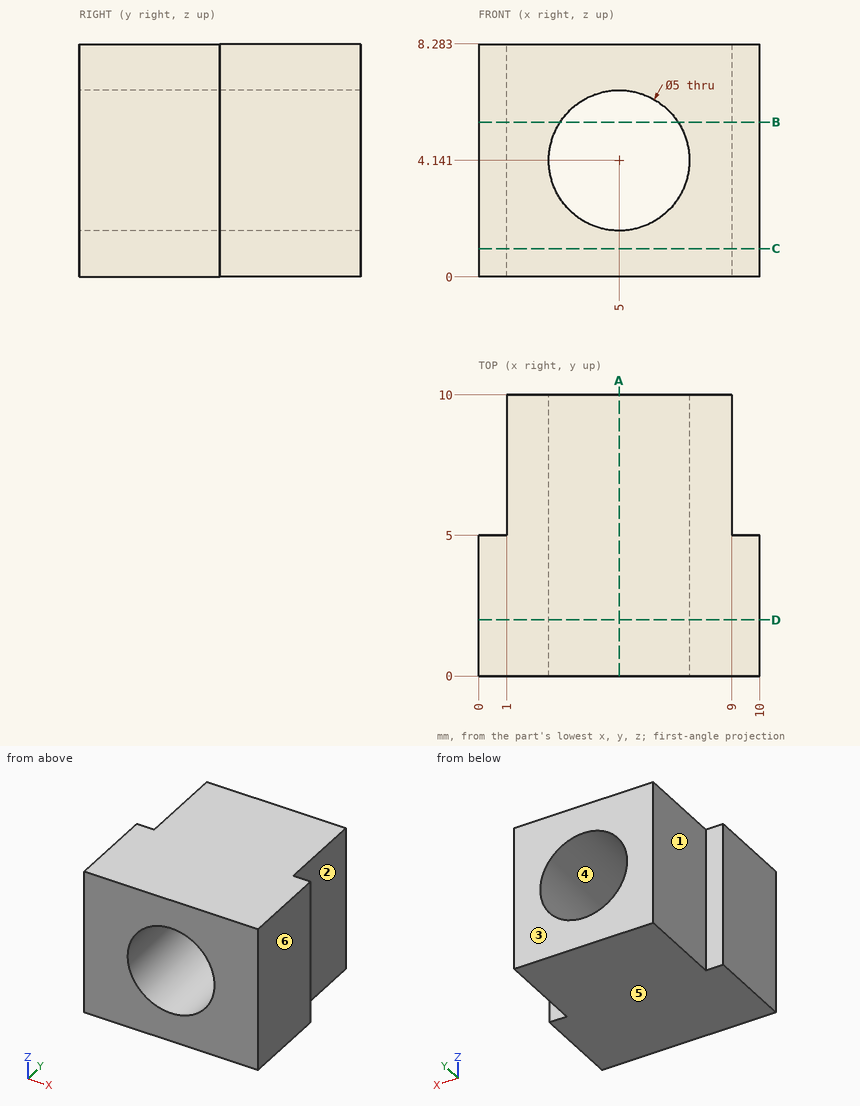
Job drawing, mm, ordinate dimensions from the low corner. One solid piece. A direction names the side the tool comes from. Give positions to 0.01 mm unless a question says otherwise; leave off trailing zeros. Order: outer loops, then holes, each group sorted by start corner. A loop starts at its lowest first (then second) coordinate and runs counter-clockwise, first axis right, second up. Notation, with made-up numbers: M 56.5,-11 L 108.5,-11 A30 ccw 108.5,27 Z; hole C 73.25,-7 d2. An arc over 180 degrees is marked long. Put each result on its own line as item: value. Start each with the question number.
(1) Pull direction Z, two halves, no side cores. Call the marked faces 4, 5 and 6: released by +Z, released by -Z, zero draft, split by the parting line, or undercut.
(2) Drill centre lines: L1, parallel to Z at x = 5, y = 2.25; L2, parallel to X at y = 4.25, z = 4; L3, parallel to Z at x = 4, y = 2.5. Where is each one in solid material? Low to high. Write a range as [from, to].
(3) Band-saw the part on C-C on z = 1. Give the cut face in (x, y).
(4) Band-saw the part on A-A on x = 5. Give the cut face in (y, z).
(5) Pin check, flat tips, straight feed: pin 1 Ø2 at (x, z) = (6.5, 4.5) entering from -Y; pin 2 Ø4 at (y, z) = (8, 2.5) entering from +X; pin 3 Ø0.8 at (x, z) = (9.5, 4) entering from +Y. Stop position of each tip, or through.
(6) Band-saw the part on B-B on z = 5.5. Give the cut face in (x, y).
(7) Tool access for the marked faces 1, 2 and 3: list every direction of +Z, -Z, +X, -X, +Y, -Y with a clear straight run to the whole face (end or side of a thin tool).
(8) Band-saw the part on D-D on y = 2. Give the cut face in (x, z).
Results below:
1. face 4: undercut
1. face 5: released by -Z
1. face 6: zero draft
2. L1: z = [0, 1.64], [6.64, 8.28]
2. L2: x = [0, 2.5], [7.5, 10]
2. L3: z = [0, 1.85], [6.43, 8.28]
3. outline: M 0,0 L 10,0 L 10,5 L 9,5 L 9,10 L 1,10 L 1,5 L 0,5 Z
4. outline: M 0,0 L 10,0 L 10,1.64 L 0,1.64 Z; M 0,6.64 L 10,6.64 L 10,8.28 L 0,8.28 Z
5. pin 1: stops at y = 0
5. pin 2: stops at x = 9
5. pin 3: stops at y = 5
6. outline: M 0,0 L 2.9,0 L 2.9,10 L 1,10 L 1,5 L 0,5 Z; M 7.1,0 L 10,0 L 10,5 L 9,5 L 9,10 L 7.1,10 Z
7. face 1: +Z, -Z, -X, +Y
7. face 2: +Z, -Z, +X, +Y
7. face 3: +Z, -Z, +X, -X, +Y
8. outline: M 0,0 L 10,0 L 10,8.28 L 0,8.28 Z; hole C 5,4.14 d5
